The model under review builds one solid part; all positions refer to its coordinate system, in mm. Give positions to 0.01 mm unless a question says otherwise; leave off trailing zeros. Loops run counter-clockwise (first coordinate to the right, second up) from the corner with the lowest first, then second, coordinate; pieces in that order, holes last. Notation, with made-up numbers: (66.25, 67.25) - (93.25, 67.25) arc R4 cw to (93.25, 71.25) - close; hole circle Ø2 at (-11, 81.5). An arc over 180 degrees is marked (long way). Return JSON: item names as keys, results as strings. Group by question number.
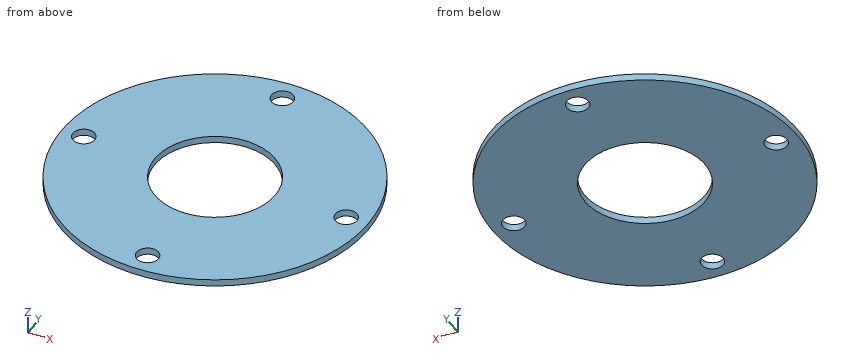
from build123d import *

# Parameters (mm, degrees)
CARRIER_REAR_START  = 32
SKETCH_1_R          = 56
SKETCH_1_R_2        = 22
CARRIER_REAR_DEPTH  = 2.5
SKETCH_2_R          = 4
THROUGH_HOLES_DEPTH = 100


with BuildPart() as part:
    # Эскиз1 → Carrier_rear (new body)
    with BuildSketch(Plane.XY.offset(CARRIER_REAR_START)):
        Circle(SKETCH_1_R)
        Circle(SKETCH_1_R_2, mode=Mode.SUBTRACT)
    extrude(amount=CARRIER_REAR_DEPTH)

    # Эскиз2 → Through_holes (cut, symmetric)
    with BuildSketch(Plane.XY):
        with Locations((48, 0)):
            Circle(SKETCH_2_R)
        with Locations((0, 48)):
            Circle(SKETCH_2_R)
        with Locations((-48, 0)):
            Circle(SKETCH_2_R)
        with Locations((0, -48)):
            Circle(SKETCH_2_R)
    extrude(amount=THROUGH_HOLES_DEPTH, both=True, mode=Mode.SUBTRACT)


solid = part.part
Item 1: Take a section at C-C (z = 32.8). State the section outline as (x, y) points, then the cut area to 3 significant figures.
Item 2: Take a section at A-A (x = 0). State the section outline as (y, z) points.
Item 3: For P1, Ø1, axis at x = -32.5, z = 33.5, coming from the +Y side, flat-tipped, find the tip position at first contact; note if it passes through.
Item 4: Take a section at D-D (y = -48). State the section outline as (x, z) points, then the cut area to 3 significant figures.
Item 5: For L1, parallel to Y at x = 0, z = 32.8; L2, parallel to X at y = 3.5, z = 32.6; L3, parallel to Y at x = 6, z = 33.8, list the stretches that pass through material, from the lowest coordinate up. Write a range as from..to.
Check sheet entries:
{
 "1": {"outline": "circle Ø112 at (0, 0); hole circle Ø8 at (-48, 0); hole circle Ø44 at (0, 0); hole circle Ø8 at (0, -48); hole circle Ø8 at (0, 48); hole circle Ø8 at (48, 0)", "area": "8,130 mm^2"},
 "2": {"outline": "(-56, 32) - (-52, 32) - (-52, 34.5) - (-56, 34.5) - close; (-44, 32) - (-22, 32) - (-22, 34.5) - (-44, 34.5) - close; (22, 32) - (44, 32) - (44, 34.5) - (22, 34.5) - close; (52, 32) - (56, 32) - (56, 34.5) - (52, 34.5) - close"},
 "3": {"P1": "stops at y = 45.96"},
 "4": {"outline": "(-28.84, 32) - (-4, 32) - (-4, 34.5) - (-28.84, 34.5) - close; (4, 32) - (28.84, 32) - (28.84, 34.5) - (4, 34.5) - close", "area": "124 mm^2"},
 "5": {"L1": "y = -56..-52, -44..-22, 22..44, 52..56", "L2": "x = -55.89..-49.94, -46.06..-21.72, 21.72..46.06, 49.94..55.89", "L3": "y = -55.68..-21.17, 21.17..55.68"}
}
